from build123d import *

# Parameters (mm, degrees)
SKETCH1_W                      = 25
SKETCH1_H                      = 38
BOSS_EXTRUDE1_DEPTH            = 6.8
SKETCH2_W                      = 23
SKETCH2_H                      = 36
CUT_EXTRUDE1_DEPTH             = 6
SKETCH2_3_W                    = 1
SKETCH2_3_H                    = 1.5
CUT_EXTRUDE2_DEPTH             = 4.8
CUT_EXTRUDE3_DEPTH             = 24.737944309
CUT_EXTRUDE3_DEPTH_BACK        = 24.737944309
SKETCH3_W                      = 6
SKETCH3_H                      = 1.2
CUT_EXTRUDE4_REACH             = 25.521
SKETCH4_W                      = 14.25
SKETCH4_H                      = 5.25
CUT_EXTRUDE4_DIRECTION_2_DEPTH = 24.521266973
SKETCH5_W                      = 1
SKETCH5_H                      = 16.8
BOSS_EXTRUDE2_DEPTH            = 6
SKETCH6_W                      = 6.5
SKETCH6_H                      = 1
CUT_EXTRUDE5_DEPTH             = 6


with BuildPart() as part:
    # Sketch1 → Boss-Extrude1 (new body)
    with BuildSketch(Plane(origin=(0, 0, 0), x_dir=(1, 0, 0), z_dir=(0, 1, 0))):
        Rectangle(SKETCH1_W, SKETCH1_H)
    extrude(amount=BOSS_EXTRUDE1_DEPTH)

    # Sketch2 → Cut-Extrude1 (cut)
    with BuildSketch(Plane(origin=(0, 6.8, 0), x_dir=(1, 0, 0), z_dir=(0, 1, 0))):
        Rectangle(SKETCH2_W, SKETCH2_H)
    extrude(amount=-CUT_EXTRUDE1_DEPTH, mode=Mode.SUBTRACT)

    # Sketch2<3> → Cut-Extrude2 (cut)
    with BuildSketch(Plane(origin=(0, 6.8, 0), x_dir=(1, 0, 0), z_dir=(0, 1, 0))):
        with Locations((-12, 17.25)):
            Rectangle(SKETCH2_3_W, SKETCH2_3_H)
        with Locations((12, 17.25)):
            Rectangle(SKETCH2_3_W, SKETCH2_3_H)
        with Locations((-12, -17.25)):
            Rectangle(SKETCH2_3_W, SKETCH2_3_H)
        with Locations((12, -17.25)):
            Rectangle(SKETCH2_3_W, SKETCH2_3_H)
    extrude(amount=-CUT_EXTRUDE2_DEPTH, mode=Mode.SUBTRACT)

    # Sketch3 → Cut-Extrude3 (cut, two sides: drawn at the far end of the back side and taken through both)
    with BuildSketch(Plane(origin=(0, 0, 0), x_dir=(0, 0, -1), z_dir=(1, 0, 0)).offset(-CUT_EXTRUDE3_DEPTH_BACK)):
        with Locations((0, 3.6)):
            Rectangle(SKETCH3_W, SKETCH3_H)
    extrude(amount=CUT_EXTRUDE3_DEPTH + CUT_EXTRUDE3_DEPTH_BACK, mode=Mode.SUBTRACT)

    # Sketch4 → Cut-Extrude4 (cut, up to next)
    with BuildSketch(Plane(origin=(0, 0.8, 0), x_dir=(1, 0, 0), z_dir=(0, 1, 0)), mode=Mode.PRIVATE) as cut_extrude4_sk1:
        with Locations((0, -11)):
            Rectangle(SKETCH4_W, SKETCH4_H)
    cut_extrude4_tool1 = extrude(cut_extrude4_sk1.sketch, amount=-CUT_EXTRUDE4_REACH, mode=Mode.PRIVATE) & part.part
    # Sketch4 → Cut-Extrude4 (cut, up to next)
    with BuildSketch(Plane(origin=(0, 0.8, 0), x_dir=(1, 0, 0), z_dir=(0, 1, 0)), mode=Mode.PRIVATE) as cut_extrude4_sk2:
        Rectangle(SKETCH4_W, SKETCH4_H)
    cut_extrude4_tool2 = extrude(cut_extrude4_sk2.sketch, amount=-CUT_EXTRUDE4_REACH, mode=Mode.PRIVATE) & part.part
    # Sketch4 → Cut-Extrude4 (cut, up to next)
    with BuildSketch(Plane(origin=(0, 0.8, 0), x_dir=(1, 0, 0), z_dir=(0, 1, 0)), mode=Mode.PRIVATE) as cut_extrude4_sk3:
        with Locations((0, 11)):
            Rectangle(SKETCH4_W, SKETCH4_H)
    cut_extrude4_tool3 = extrude(cut_extrude4_sk3.sketch, amount=-CUT_EXTRUDE4_REACH, mode=Mode.PRIVATE) & part.part
    add(cut_extrude4_tool1.solids().sort_by_distance((0, 0.8, 11))[0], mode=Mode.SUBTRACT)
    add(cut_extrude4_tool2.solids().sort_by_distance((0, 0.8, 0))[0], mode=Mode.SUBTRACT)
    add(cut_extrude4_tool3.solids().sort_by_distance((0, 0.8, -11))[0], mode=Mode.SUBTRACT)

    # Sketch4 → Cut-Extrude4 direction 2 (cut)
    with BuildSketch(Plane(origin=(0, 0.8, 0), x_dir=(1, 0, 0), z_dir=(0, 1, 0))):
        with Locations((0, -11)):
            Rectangle(SKETCH4_W, SKETCH4_H)
        Rectangle(SKETCH4_W, SKETCH4_H)
        with Locations((0, 11)):
            Rectangle(SKETCH4_W, SKETCH4_H)
    extrude(amount=CUT_EXTRUDE4_DIRECTION_2_DEPTH, mode=Mode.SUBTRACT)

    # Sketch5 → Boss-Extrude2 (add)
    with BuildSketch(Plane(origin=(0, 0.8, 0), x_dir=(1, 0, 0), z_dir=(0, 1, 0))):
        with Locations((-9, 0)):
            Rectangle(SKETCH5_W, SKETCH5_H)
        with Locations((9, 0)):
            Rectangle(SKETCH5_W, SKETCH5_H)
    extrude(amount=BOSS_EXTRUDE2_DEPTH)

    # Sketch6 → Cut-Extrude5 (cut)
    with BuildSketch(Plane(origin=(0, 6.8, 0), x_dir=(1, 0, 0), z_dir=(0, 1, 0))):
        with Locations((0, -18.5)):
            Rectangle(SKETCH6_W, SKETCH6_H)
    extrude(amount=-CUT_EXTRUDE5_DEPTH, mode=Mode.SUBTRACT)


solid = part.part
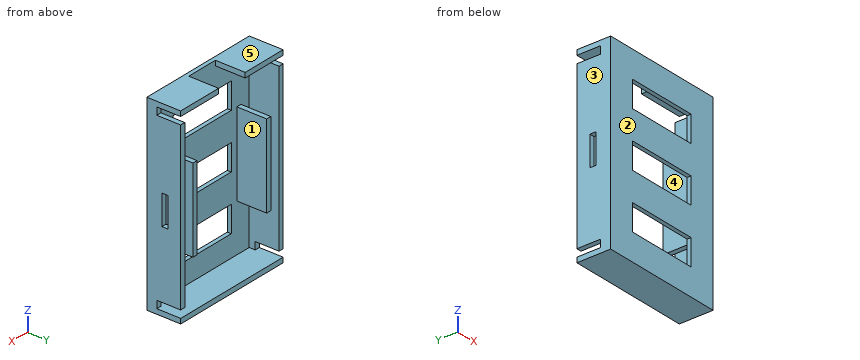
Read the model definition and answer for the solid it produces. Units are mm, in the model's axes. Face numbers are marked on the shaded views. A direction names the side the tool comes from. Round coordinates to 2 decimals unless told otherwise and drop trailing zeros. Write each loop counter-clockwise with the first axis right and the second up, starting at its lowest first coordinate (ties: lowest second). Pieces come first, ordered by that corner, then holes. Notation, with made-up numbers: (-27, -17) - (26, -17) arc R20 cw to (26, -11) - close; hole circle Ø10 at (70.25, 71). An arc over 180 degrees is marked (long way). Use a Markdown table: item, result.
(1) The mould has two halves that part along X. Classify the marked faces 1, 2 and 3: released by +X, released by -X, zero draft, split by the parting line, or undercut.
Reported:
| item | result |
|---|---|
| face 1 | undercut |
| face 2 | zero draft |
| face 3 | released by -X |
(2) The part is cut by section A-A (x = 1.5). Write down the section's boundary in (y, z) (3 decimals), then the cut area to 3 significant figures.
Reported:
| item | result |
|---|---|
| outline | (0, -19) - (6.8, -19) - (6.8, -18) - (0.8, -18) - (0.8, -13.625) - (0, -13.625) - close; (0, -8.375) - (0.8, -8.375) - (0.8, -2.625) - (0, -2.625) - close; (0, 2.625) - (0.8, 2.625) - (0.8, 8.375) - (0, 8.375) - close; (0, 13.625) - (0.8, 13.625) - (0.8, 19) - (0, 19) - close |
| area | 23.8 mm2 |
(3) Straight lines are drawn through the part: line 1 along X through (y, z) = (3, -5); line 2 along Z through (x, y) = (-9.25, 4); line 3 along Z through (x, y) = (-4, 6). For each, find the intervals that lie inside material, in ascending order. Write a range as [from, to].
Reported:
| item | result |
|---|---|
| line 1 | [-12.5, -11.5], [-9.5, -8.5], [8.5, 9.5], [11.5, 12.5] |
| line 2 | [-19, -18], [-8.4, 8.4], [18, 19] |
| line 3 | [-19, -18], [18, 19] |
(4) Which of the six approach directions +Z, -Z, +X, -X, +Y, -Y give full straight-line access (tool end or side, diameter ignored) to the marked faces 4 and 5?
Reported:
| item | result |
|---|---|
| face 4 | +Y |
| face 5 | +Z, +X, -X, +Y, -Y |
(5) Each of these flat-tipped pins is pushed along its axis until it touches: pin 1 Ø12 at (x, z) = (0.5, -4.5) entering from +Y; pin 2 Ø1.5 at (x, y) = (-2, 4) entering from +Z. Where does it stop, or does it pass through?
Reported:
| item | result |
|---|---|
| pin 1 | y = 0.8 |
| pin 2 | z = -18 |
(6) The part is cut by section C-C (z = -2). Write down the section's boundary in (x, y) (3 decimals).
Reported:
| item | result |
|---|---|
| outline | (-12.5, 0) - (-7.125, 0) - (-7.125, 0.8) - (-8.5, 0.8) - (-8.5, 6.8) - (-9.5, 6.8) - (-9.5, 0.8) - (-11.5, 0.8) - (-11.5, 3) - (-12.5, 3) - close; (-12.5, 4.2) - (-11.5, 4.2) - (-11.5, 6.8) - (-12.5, 6.8) - close; (7.125, 0) - (12.5, 0) - (12.5, 3) - (11.5, 3) - (11.5, 0.8) - (9.5, 0.8) - (9.5, 6.8) - (8.5, 6.8) - (8.5, 0.8) - (7.125, 0.8) - close; (11.5, 4.2) - (12.5, 4.2) - (12.5, 6.8) - (11.5, 6.8) - close |
(7) The part is cut by section D-D (x = 9). Write down the section's boundary in (y, z).
Reported:
| item | result |
|---|---|
| outline | (0, -19) - (6.8, -19) - (6.8, -18) - (0.8, -18) - (0.8, -8.4) - (6.8, -8.4) - (6.8, 8.4) - (0.8, 8.4) - (0.8, 18) - (6.8, 18) - (6.8, 19) - (0, 19) - close |
(8) The part is cut by section B-B (y = 6). Write down the section's boundary in (x, z), then the cut area to 3 significant figures.
Reported:
| item | result |
|---|---|
| outline | (-12.5, -19) - (12.5, -19) - (12.5, -18) - (-12.5, -18) - close; (-12.5, -16.5) - (-11.5, -16.5) - (-11.5, 16.5) - (-12.5, 16.5) - close; (-12.5, 18) - (-3.25, 18) - (-3.25, 19) - (-12.5, 19) - close; (-9.5, -8.4) - (-8.5, -8.4) - (-8.5, 8.4) - (-9.5, 8.4) - close; (3.25, 18) - (12.5, 18) - (12.5, 19) - (3.25, 19) - close; (8.5, -8.4) - (9.5, -8.4) - (9.5, 8.4) - (8.5, 8.4) - close; (11.5, -16.5) - (12.5, -16.5) - (12.5, 16.5) - (11.5, 16.5) - close |
| area | 143 mm2 |
